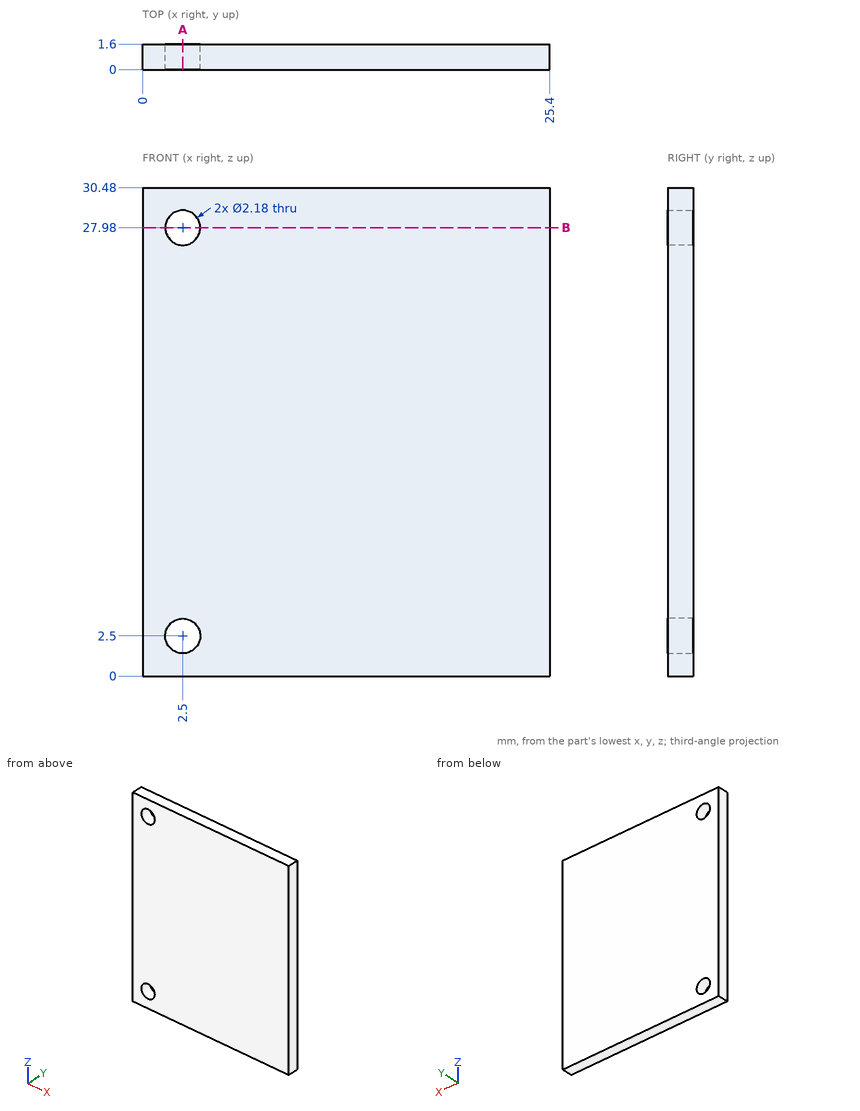
Can you work these out from the drawing? Everything is in mm from the part's minimum corner. Coordinates: 2 decimals unless noted, no trailing zeros. Write each loop counter-clockwise with the first axis right and the second up, starting at its lowest first coordinate (ties: lowest second). Pieces come first, ordered by that corner, then holes. Notation, with made-up numbers: (24, -22) -> (43, -22) arc R24 ccw to (43, 17) -> close; hole circle Ø11 at (-1, 29.5). An arc over 180 degrees is marked (long way). Write each question's results on one line, items separated by ' | '. Start each with the question number.
Q1. I'm going to push a flat-ended pin straight in: pin 1 (2 mm diameter, centred on x = 2.5, z = 27.98, fed in from -Y). Where does the tip first touch, or does it pass through?
Q2. Imagine slicing it at A-A (x = 2.5). Write out the boundary of the cut face in (y, z), then the cut area to 3 significant figures.
Q3. If I drill on probe 1 along X at (y, z) = (1.25, 2.5), over which ranges is the centre line in solid material (lowest first)?
Q4. Imagine slicing it at B-B (z = 27.98). Write out the boundary of the cut face in (x, y).
Taken from the geometry:
1) pin 1: passes through
2) outline: (0, 0) -> (1.6, 0) -> (1.6, 1.41) -> (0, 1.41) -> close; (0, 3.59) -> (1.6, 3.59) -> (1.6, 26.89) -> (0, 26.89) -> close; (0, 29.07) -> (1.6, 29.07) -> (1.6, 30.48) -> (0, 30.48) -> close | area: 41.8 mm^2
3) probe 1: x = 0 to 1.41, 3.59 to 25.4
4) outline: (0, 0) -> (1.41, 0) -> (1.41, 1.6) -> (0, 1.6) -> close; (3.59, 0) -> (25.4, 0) -> (25.4, 1.6) -> (3.59, 1.6) -> close
